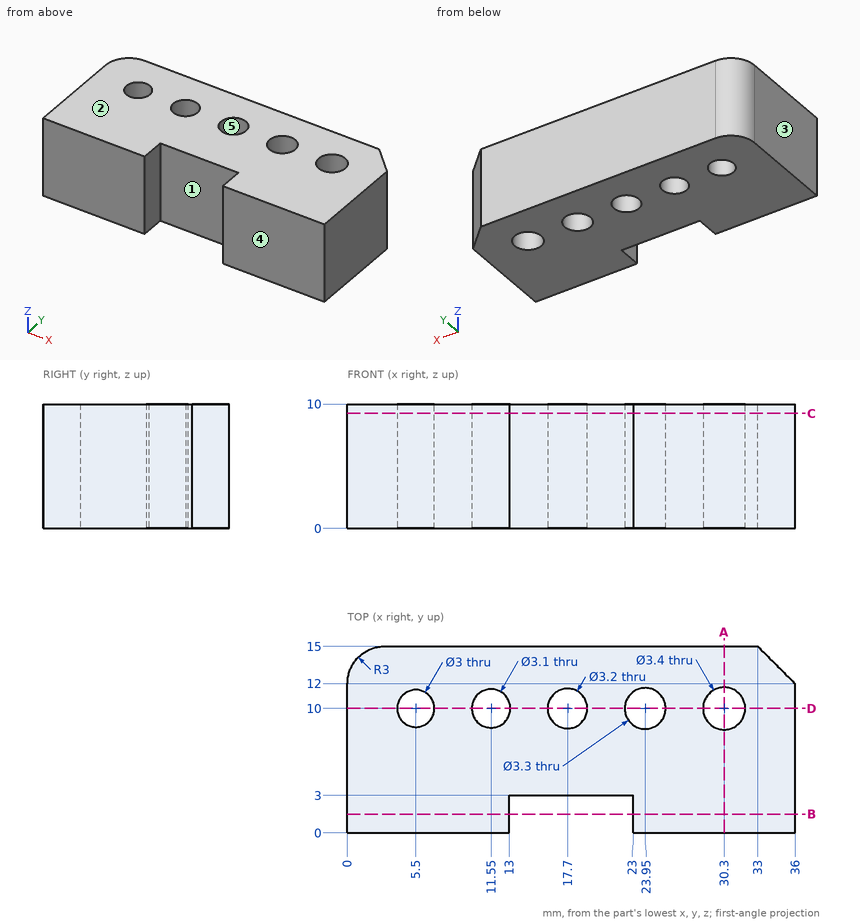
Check sheet for the drawn part. Datum: minimum x, y, z corner. Units: mm. A direction names the side the tool comes from. Give positions to 0.01 mm unless a question says otherwise; leave off trailing zeros. Order: outer loops, then holes, each group sorted by start corner. A loop starts at its lowest first (then second) coordinate and runs counter-clockwise, first axis right, second up. Notation, with made-up numbers: (67, -30) - (108, -30) arc R15 ccw to (108, -11) - close; hole circle Ø6 at (29, -30.5). An arc over 180 degrees is marked (long way). Answer in a Markdown table with one row per item. Add a question column.
Q1. Mould release check, pull along X, two halves, no side actions. Record for the marked faces 3, 4 and 5: pulls with the +X half, pulls with the -X half, needs draft (parallel to the pull), parting line crosses it, or undercut.
Q2. Cross-section at D-D, the plane y = 10. Enter the section's corners in (x, z).
Q3. Material ranges on probe 1 along Y at (x, z) = (17.7, 4); probe 2 along X at (y, z) = (2.25, 7.5); probe 3 along Y at (x, z) = (5.5, 5.25), recorded low to high. Write a range as from..to.
Q4. Cross-section at B-B, the plane y = 1.5. Enter the section's corners in (x, z).
Q5. Tool access check on the marked faces 1 and 2. Record the directions out of +Z, -Z, +X, -X, +Y, -Y that give a thin tool (end or side, any length) a straight path to the whole face; none if there is none.
Q6. Cross-section at C-C, the plane z = 9.25. Enter the section's corners in (x, y), then the cut area to 3 significant figures.
Q7. Cross-section at A-A, the plane x = 30.3. Enter the section's corners in (y, z).
Check values:
| question | item | result |
|---|---|---|
| 1 | face 3 | pulls with the -X half |
| 1 | face 4 | needs draft |
| 1 | face 5 | undercut |
| 2 | outline | (0, 0) - (4, 0) - (4, 10) - (0, 10) - close; (7, 0) - (10, 0) - (10, 10) - (7, 10) - close; (13.1, 0) - (16.1, 0) - (16.1, 10) - (13.1, 10) - close; (19.3, 0) - (22.3, 0) - (22.3, 10) - (19.3, 10) - close; (25.6, 0) - (28.6, 0) - (28.6, 10) - (25.6, 10) - close; (32, 0) - (36, 0) - (36, 10) - (32, 10) - close |
| 3 | probe 1 | y = 3..8.4, 11.6..15 |
| 3 | probe 2 | x = 0..13, 23..36 |
| 3 | probe 3 | y = 0..8.5, 11.5..15 |
| 4 | outline | (0, 0) - (13, 0) - (13, 10) - (0, 10) - close; (23, 0) - (36, 0) - (36, 10) - (23, 10) - close |
| 5 | face 1 | +Z, -Z, -Y |
| 5 | face 2 | +Z, +X, -X, +Y, -Y |
| 6 | outline | (0, 0) - (13, 0) - (13, 3) - (23, 3) - (23, 0) - (36, 0) - (36, 12) - (33, 15) - (3, 15) arc R3 ccw to (0, 12) - close; hole circle Ø3 at (5.5, 10); hole circle Ø3.1 at (11.55, 10); hole circle Ø3.2 at (17.7, 10); hole circle Ø3.3 at (23.95, 10); hole circle Ø3.4 at (30.3, 10) |
| 6 | area | 463 mm^2 |
| 7 | outline | (0, 0) - (8.3, 0) - (8.3, 10) - (0, 10) - close; (11.7, 0) - (15, 0) - (15, 10) - (11.7, 10) - close |
